Part model, mm, in its own coordinate system. A direction names the side the tool comes from. Coordinates: 2 decimals unless noted, no trailing zeros. Use a Markdown table: item, result. Add a question column.
1) Tool access for faces 1 (the face through (103.114, 24, -42)), 2 (the face through (103.114, 24, 42)), 3 (the face through (-103.114, 24, 42)), 4 (the face through (103, -5.71, 0)): list every direction of +Z, -Z, +X, -X, +Y, -Y with a clear straight run to the whole face (end or side of a thin tool).
2) Wall check: L1, parallel to Z at x = 75, y = 13.5; L2, parallel to X at y = 22, z = -35; L3, parallel to Y at x = -31, z = -39. Give the ranges that are in metal, low to high. Write a range as [from, to].
3) Drop flat-ended pins along their axis: P1, Ø8, axis at x = 18, y = -2, coming from the +Z side; P2, Ø5, axis at x = 46, z = -39.5, coming from the +Y side; P3, Ø1, axis at y = 33, z = 34, coming from the +X side. Give the stop position or say it passes through.
4) Two-plate mould, pull along Z, no slides. Class faces 5 (the face through (-1, 32.29, -1)), 6 (the face through (-1, 24, 63.744)), 7 (the face through (-103.114, 24, -42)): +Z half, -Z half, draft (parallel to the pull), parting line (faces both ways), or undercut.
```python
from build123d import *

# Parameters (mm, degrees)
SKETCH1_W           = 218.44
SKETCH1_H           = 139.7
BOSS_EXTRUDE1_DEPTH = 34.29
SKETCH2_W           = 238.44
SKETCH2_H           = 159.7
SKETCH2_W_2         = 198.44
SKETCH2_H_2         = 119.7
CUT_EXTRUDE1_DEPTH  = 172.72
CUT_EXTRUDE1_TAPER  = 3.25
SKETCH3_W           = 206.22850923
SKETCH3_H           = 127.48850923
BOSS_EXTRUDE2_DEPTH = 20
BOSS_EXTRUDE3_START = -20
SKETCH4_W           = 40
SKETCH4_H           = 40
BOSS_EXTRUDE3_DEPTH = 22
CUT_EXTRUDE2_DEPTH  = 2


with BuildPart() as part:
    # Sketch1 → Boss-Extrude1 (new body, symmetric)
    with BuildSketch(Plane(origin=(0, 0, 0), x_dir=(1, 0, 0), z_dir=(0, 1, 0))):
        Rectangle(SKETCH1_W, SKETCH1_H)
    extrude(amount=BOSS_EXTRUDE1_DEPTH, both=True)

    # Sketch2 → Cut-Extrude1 (cut)
    with BuildSketch(Plane.XZ.offset(34.29)):
        Rectangle(SKETCH2_W, SKETCH2_H)
        Rectangle(SKETCH2_W_2, SKETCH2_H_2, mode=Mode.SUBTRACT)
    extrude(amount=-CUT_EXTRUDE1_DEPTH, taper=CUT_EXTRUDE1_TAPER, mode=Mode.SUBTRACT)

    # Sketch3 → Boss-Extrude2 (add)
    with BuildSketch(Plane(origin=(0, 34.29, 0), x_dir=(1, 0, 0), z_dir=(0, 1, 0))):
        Rectangle(SKETCH3_W, SKETCH3_H)
    extrude(amount=-BOSS_EXTRUDE2_DEPTH)

    # Sketch4 → Boss-Extrude3 (add)
    with BuildSketch(Plane(origin=(103.114254615, 0, 0), x_dir=(0, 0, -1), z_dir=(1, 0, 0)).offset(BOSS_EXTRUDE3_START)):
        with Locations((0, 14.29)):
            Rectangle(SKETCH4_W, SKETCH4_H)
    boss_extrude3 = extrude(amount=BOSS_EXTRUDE3_DEPTH)

    # Mirror1: Boss-Extrude3 across plane
    add(boss_extrude3.mirror(Plane(origin=(0, 0, 0), x_dir=(0, 0, 1), z_dir=(1, 0, 0))))

    # Sketch5 → Cut-Extrude2 (cut)
    with BuildSketch(Plane(origin=(0, 34.29, 0), x_dir=(1, 0, 0), z_dir=(0, 1, 0))):
        Polygon((-88.114254615, 48.744254615), (-88.114254615, 5), (-90.114254615, 5), (-90.114254615, -5), (-88.114254615, -5), (-88.114254615, -48.744254615), (88.114254615, -48.744254615), (88.114254615, -5), (90.114254615, -5), (90.114254615, 5), (88.114254615, 5), (88.114254615, 48.744254615), align=None)
    extrude(amount=-CUT_EXTRUDE2_DEPTH, mode=Mode.SUBTRACT)


solid = part.part
```
Results are:
| question | item | result |
|---|---|---|
| 1 | face 1 | -Z, +X, +Y, -Y |
| 1 | face 2 | +Z, +X, +Y, -Y |
| 1 | face 3 | +Z, -X, +Y, -Y |
| 1 | face 4 | +Z, -Z, +X, -Y |
| 2 | L1 | [-62.56, 62.56] |
| 2 | L2 | [-103.11, 103.11] |
| 2 | L3 | [-34.29, 32.29] |
| 3 | P1 | z = 61.91 |
| 3 | P2 | y = 32.29 |
| 3 | P3 | x = 103.11 |
| 4 | face 5 | undercut |
| 4 | face 6 | +Z half |
| 4 | face 7 | draft |
